Could you check a few things on this model? Use its own coordinates, in mm. Give positions to 0.01 mm unless a question says otherwise; leave off trailing zeros. Write each loop counter-clockwise with the first axis right and the second up, starting at its lowest first coordinate (ties: lowest second). Pieces come first, ordered by that corner, then holes. Notation, with made-up numbers: (25.25, 67.5) - (59.25, 67.5) arc R21 ccw to (59.25, 75.5) - close; hole circle Ø2 at (-9.75, -27.5). An arc over 180 degrees is marked (long way). Write item = value, one per line.
from build123d import *

# Parameters (mm, degrees)
BOSS_EXTRUDE1_DEPTH                    = 20
CBORE_FOR_M8_HEX_HEAD_BOLT1_AT_2_COUNT = 2
CBORE_FOR_M8_HEX_HEAD_BOLT1_AT_2_PITCH = 45
CBORE_FOR_M8_HEX_HEAD_BOLT1_AT_3_COUNT = 2
CBORE_FOR_M8_HEX_HEAD_BOLT1_AT_3_PITCH = 1307.399809271
CBORE_FOR_M8_HEX_HEAD_BOLT1_AT_4_COUNT = 2
CBORE_FOR_M8_HEX_HEAD_BOLT1_AT_4_PITCH = 90
CBORE_FOR_M6_HEX_HEAD_BOLT1_AT_2_COUNT = 2
CBORE_FOR_M6_HEX_HEAD_BOLT1_AT_2_PITCH = 100
CBORE_FOR_M6_HEX_HEAD_BOLT1_AT_3_COUNT = 2
CBORE_FOR_M6_HEX_HEAD_BOLT1_AT_3_PITCH = 199.997125624
CHAMFER1_SIZE                          = 1
CHAMFER2_SIZE                          = 1
CUT_EXTRUDE14_DEPTH                    = 7
SKETCH49_R                             = 13
CUT_EXTRUDE15_DEPTH                    = 529.16388983
FILLET1_SIZE                           = 5


with BuildPart() as part:
    # Sketch1 → Boss-Extrude1 (new body)
    with BuildSketch(Plane.XY):
        with BuildLine():
            Line((-495, 33.117706736), (-495, 178.117706736))
            ThreePointArc((-495, 178.117706736), (-493.535533906, 181.653240642), (-490, 183.117706736))
            Line((-490, 183.117706736), (-400, 183.117706736))
            Line((-400, 183.117706736), (-400, 138.117706736))
            Line((-400, 138.117706736), (0, 138.117706736))
            Line((0, 138.117706736), (400, 138.117706736))
            Line((400, 138.117706736), (400, 183.117706736))
            Line((400, 183.117706736), (490, 183.117706736))
            ThreePointArc((490, 183.117706736), (493.535533906, 181.653240642), (495, 178.117706736))
            Line((495, 178.117706736), (495, 33.117706736))
            ThreePointArc((495, 33.117706736), (483.284271247, 4.833435489), (455, -6.882293264))
            Line((455, -6.882293264), (315, -6.882293264))
            ThreePointArc((315, -6.882293264), (300.857864376, -1.024428888), (295, 13.117706736))
            Line((295, 13.117706736), (295, 38.117706736))
            ThreePointArc((295, 38.117706736), (292.071067812, 45.188774548), (285, 48.117706736))
            Line((285, 48.117706736), (-285, 48.117706736))
            ThreePointArc((-285, 48.117706736), (-292.071067812, 45.188774548), (-295, 38.117706736))
            Line((-295, 38.117706736), (-295, 13.117706736))
            ThreePointArc((-295, 13.117706736), (-300.857864376, -1.024428888), (-315, -6.882293264))
            Line((-315, -6.882293264), (-455, -6.882293264))
            ThreePointArc((-455, -6.882293264), (-483.284271247, 4.833435489), (-495, 33.117706736))
        make_face()
    extrude(amount=BOSS_EXTRUDE1_DEPTH)

    # Sketch6 → CBORE for M8 Hex Head Bolt1 (revolve, cut)
    with BuildSketch(Plane(origin=(-422.5, 160.617706736, 20), x_dir=(0, -1, 0), z_dir=(1, 0, 0))):
        Polygon((0, 0), (0, 20), (4.5, 20), (4.5, 5.3), (9.0055, 5.3), (9.0055, 0.025), (9.0305, 0), align=None)
    cbore_for_m8_hex_head_bolt1 = revolve(axis=Axis((-422.5, 160.617706736, 26.35), (0, 0, -1)), mode=Mode.SUBTRACT)

    # CBORE for M8 Hex Head Bolt1 at 2: CBORE for M8 Hex Head Bolt1 ×2
    with Locations(*[(0, -i * CBORE_FOR_M8_HEX_HEAD_BOLT1_AT_2_PITCH, 0) for i in range(1, CBORE_FOR_M8_HEX_HEAD_BOLT1_AT_2_COUNT)]):
        add(cbore_for_m8_hex_head_bolt1, mode=Mode.SUBTRACT)

    # CBORE for M8 Hex Head Bolt1 at 3: CBORE for M8 Hex Head Bolt1 ×2
    with Locations(*[Vector(-0.7034023303245859, 0.710791925737724, 0) * (i * CBORE_FOR_M8_HEX_HEAD_BOLT1_AT_3_PITCH) for i in range(1, CBORE_FOR_M8_HEX_HEAD_BOLT1_AT_3_COUNT)]):
        add(cbore_for_m8_hex_head_bolt1, mode=Mode.SUBTRACT)

    # CBORE for M8 Hex Head Bolt1 at 4: CBORE for M8 Hex Head Bolt1 ×2
    with Locations(*[(0, -i * CBORE_FOR_M8_HEX_HEAD_BOLT1_AT_4_PITCH, 0) for i in range(1, CBORE_FOR_M8_HEX_HEAD_BOLT1_AT_4_COUNT)]):
        add(cbore_for_m8_hex_head_bolt1, mode=Mode.SUBTRACT)

    # Mirror1: CBORE for M8 Hex Head Bolt1 across plane
    add(cbore_for_m8_hex_head_bolt1.mirror(Plane(origin=(0, 0, 0), x_dir=(0, 0, 1), z_dir=(1, 0, 0))), mode=Mode.SUBTRACT)

    # Mirror1 copy 1 sketch → Mirror1 copy 1 (revolve, cut)
    with BuildSketch(Plane(origin=(422.5, 115.617706736, 20), x_dir=(0, -1, 0), z_dir=(-1, 0, 0))):
        Polygon((0, 0), (0, -20), (4.5, -20), (4.5, -5.3), (9.0055, -5.3), (9.0055, -0.025), (9.0305, 0), align=None)
    revolve(axis=Axis((422.5, 115.617706736, 26.35), (0, 0, 1)), mode=Mode.SUBTRACT)

    # Mirror1 copy 2 sketch → Mirror1 copy 2 (revolve, cut)
    with BuildSketch(Plane(origin=(1342.128072507, 1089.906934877, 20), x_dir=(0, -1, 0), z_dir=(-1, 0, 0))):
        Polygon((0, 0), (0, -20), (4.5, -20), (4.5, -5.3), (9.0055, -5.3), (9.0055, -0.025), (9.0305, 0), align=None)
    revolve(axis=Axis((1342.128072507, 1089.906934877, 26.35), (0, 0, 1)), mode=Mode.SUBTRACT)

    # Mirror1 copy 3 sketch → Mirror1 copy 3 (revolve, cut)
    with BuildSketch(Plane(origin=(422.5, 70.617706736, 20), x_dir=(0, -1, 0), z_dir=(-1, 0, 0))):
        Polygon((0, 0), (0, -20), (4.5, -20), (4.5, -5.3), (9.0055, -5.3), (9.0055, -0.025), (9.0305, 0), align=None)
    revolve(axis=Axis((422.5, 70.617706736, 26.35), (0, 0, 1)), mode=Mode.SUBTRACT)

    # Sketch8 → CBORE for M6 Hex Head Bolt1 (revolve, cut)
    with BuildSketch(Plane(origin=(-385, 115.617706736, 20), x_dir=(0, -1, 0), z_dir=(1, 0, 0))):
        Polygon((0, 0), (0, 20.001), (3.3, 20.001), (3.3, 4), (7.2735, 4), (7.2735, 0.025), (7.2985, 0), align=None)
    cbore_for_m6_hex_head_bolt1 = revolve(axis=Axis((-385, 115.617706736, 26.35), (0, 0, -1)), mode=Mode.SUBTRACT)

    # CBORE for M6 Hex Head Bolt1 at 2: CBORE for M6 Hex Head Bolt1 ×2
    with Locations(*[(i * CBORE_FOR_M6_HEX_HEAD_BOLT1_AT_2_PITCH, 0, 0) for i in range(1, CBORE_FOR_M6_HEX_HEAD_BOLT1_AT_2_COUNT)]):
        add(cbore_for_m6_hex_head_bolt1, mode=Mode.SUBTRACT)

    # CBORE for M6 Hex Head Bolt1 at 3: CBORE for M6 Hex Head Bolt1 ×2
    with Locations(*[(i * CBORE_FOR_M6_HEX_HEAD_BOLT1_AT_3_PITCH, 0, 0) for i in range(1, CBORE_FOR_M6_HEX_HEAD_BOLT1_AT_3_COUNT)]):
        add(cbore_for_m6_hex_head_bolt1, mode=Mode.SUBTRACT)

    # Mirror2: CBORE for M6 Hex Head Bolt1 across plane
    add(cbore_for_m6_hex_head_bolt1.mirror(Plane(origin=(0, 0, 0), x_dir=(0, 0, 1), z_dir=(1, 0, 0))), mode=Mode.SUBTRACT)

    # Mirror2 copy 1 sketch → Mirror2 copy 1 (revolve, cut)
    with BuildSketch(Plane(origin=(285, 115.617706736, 20), x_dir=(0, -1, 0), z_dir=(-1, 0, 0))):
        Polygon((0, 0), (0, -20.001), (3.3, -20.001), (3.3, -4), (7.2735, -4), (7.2735, -0.025), (7.2985, 0), align=None)
    revolve(axis=Axis((285, 115.617706736, 26.35), (0, 0, 1)), mode=Mode.SUBTRACT)

    # Mirror2 copy 2 sketch → Mirror2 copy 2 (revolve, cut)
    with BuildSketch(Plane(origin=(185.002874376, 115.617706736, 20), x_dir=(0, -1, 0), z_dir=(-1, 0, 0))):
        Polygon((0, 0), (0, -20.001), (3.3, -20.001), (3.3, -4), (7.2735, -4), (7.2735, -0.025), (7.2985, 0), align=None)
    revolve(axis=Axis((185.002874376, 115.617706736, 26.35), (0, 0, 1)), mode=Mode.SUBTRACT)

    # Chamfer1
    chamfer1_edges = [part.edges().sort_by_distance(p)[0] for p in [
        (292.071067812, 45.188774548, 20),
        (295, 25.617706736, 20),
        (300.857864376, -1.024428888, 20),
        (385, -6.882293264, 20),
        (483.284271247, 4.833435489, 20),
        (495, 105.617706736, 20),
        (493.535533906, 181.653240642, 20),
        (445, 183.117706736, 20),
        (-292.071067812, 45.188774548, 20),
        (-445, 183.117706736, 20),
        (-493.535533906, 181.653240642, 20),
        (-495, 105.617706736, 20),
        (-483.284271247, 4.833435489, 20),
        (-385, -6.882293264, 20),
        (-300.857864376, -1.024428888, 20),
        (-295, 25.617706736, 20),
        (0, 48.117706736, 20),
    ]]
    chamfer(chamfer1_edges, length=CHAMFER1_SIZE)

    # Chamfer2
    chamfer2_edges = [part.edges().sort_by_distance(p)[0] for p in [
        (-295, 25.617706736, 0),
        (-300.857864376, -1.024428888, 0),
        (-385, -6.882293264, 0),
        (-483.284271247, 4.833435489, 0),
        (-495, 105.617706736, 0),
        (-493.535533906, 181.653240642, 0),
        (-445, 183.117706736, 0),
        (445, 183.117706736, 0),
        (493.535533906, 181.653240642, 0),
        (495, 105.617706736, 0),
        (483.284271247, 4.833435489, 0),
        (385, -6.882293264, 0),
        (300.857864376, -1.024428888, 0),
        (295, 25.617706736, 0),
        (292.071067812, 45.188774548, 0),
        (0, 48.117706736, 0),
        (-292.071067812, 45.188774548, 0),
    ]]
    chamfer(chamfer2_edges, length=CHAMFER2_SIZE)

    # Sketch16 → Cut-Extrude14 (cut)
    with BuildSketch(Plane.XY.offset(20)):
        Polygon((-375.773169187, 78.117706736), (-344.229306438, 78.117706736), (-339, 72.886119668), (-339, 41.351758145), (-344.226830813, 36.117706736), (-375.770693562, 36.117706736), (-381, 41.349293804), (-381, 72.883655327), align=None)
    cut_extrude14 = extrude(amount=-CUT_EXTRUDE14_DEPTH, mode=Mode.SUBTRACT)

    # Sketch49 → Cut-Extrude15 (cut, through all)
    with BuildSketch(Plane.XY.offset(20)):
        with Locations((-360, 57.117706736)):
            Circle(SKETCH49_R)
    cut_extrude15 = extrude(amount=-CUT_EXTRUDE15_DEPTH, mode=Mode.SUBTRACT)

    # Mirror3: Cut-Extrude14, Cut-Extrude15 across plane
    add(cut_extrude14.mirror(Plane(origin=(0, 0, 0), x_dir=(0, 0, 1), z_dir=(1, 0, 0))), mode=Mode.SUBTRACT)
    add(cut_extrude15.mirror(Plane(origin=(0, 0, 0), x_dir=(0, 0, 1), z_dir=(1, 0, 0))), mode=Mode.SUBTRACT)

    # Fillet1
    fillet1_edges = [part.edges().sort_by_distance(p)[0] for p in [
        (-400, 138.117706736, 10),
        (-400, 183.117706736, 10),
        (400, 183.117706736, 10),
        (400, 138.117706736, 10),
    ]]
    chamfer(fillet1_edges, length=FILLET1_SIZE)


solid = part.part
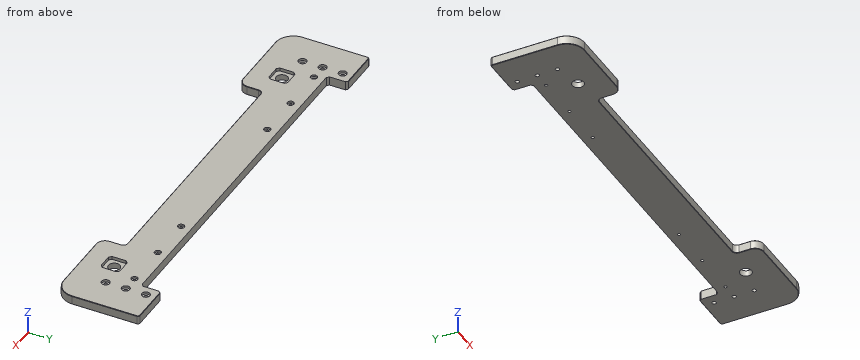
1. For pin 1 (23.5 mm diameter, centred on x = 422.5, y = 160.62, fed in from -Z); pin 2 (14.5 mm diameter, centred on x = -422.5, y = 115.62, fed in from +Z); pin 3 (8.5 mm diameter, centred on x = 185, y = 115.62, fed in from +Z); pin 4 (1 mm diameter, centred on x = 170.5, z = 3.5, fed in from -Y), each with a flat end and sliding along its axis, tell me the tip position at first contact or that it passes through.
Filled sheet:
pin_1 = 0
pin_2 = 14.7
pin_3 = 16
pin_4 = 48.12
2. If we section it at A-A, the plane x = -360: Please give me the cut outline in (y, z), and give its area (3 significant figures).
Filled sheet:
outline = (-6.88, 1) - (-5.88, 0) - (44.12, 0) - (44.12, 13) - (36.12, 13) - (36.12, 20) - (-5.88, 20) - (-6.88, 19) - close; (70.12, 0) - (138.12, 0) - (138.12, 20) - (78.12, 20) - (78.12, 13) - (70.12, 13) - close
area = 2,270 mm2
3. If we section it at B-B, the plane x = -217: Please give me the cut outline in (y, z).
Filled sheet:
outline = (48.12, 1) - (49.12, 0) - (138.12, 0) - (138.12, 20) - (49.12, 20) - (48.12, 19) - close
4. I need wall thicknesses on line 1 (X direction, y = 72, z = 18); line 2 (Y direction, x = -422.5, z = 18); line 3 (X direction, y = 58, z = 9). Which ranges of each line are inside material? Lowest first, please.
Filled sheet:
line_1 = -495 to -431.4, -413.6 to -381, -339 to 339, 381 to 413.6, 431.4 to 495
line_2 = -6.88 to 61.61, 79.62 to 106.61, 124.62 to 151.61, 169.62 to 183.12
line_3 = -495 to -372.97, -347.03 to 347.03, 372.97 to 495
